Can you work these out from the model? Positions are in its coordinate system, mm. A direction names the side the tool comes from. Coordinates: 2 decimals unless noted, no trailing zeros. Write each loop counter-clockwise with the first axis right and the second up, starting at its lowest first coordinate (ties: lowest second). Pieces come first, ordered by that corner, then holes. Notation, with made-up numbers: (64, 25.5) - (104, 25.5) arc R19 ccw to (104, 31.5) - close; hole circle Ø8 at (-4.75, 21). An arc over 180 degrees is marked (long way). Use one line per item in the form item = value. Start each with the question number.
(1) If I drill on probe 1 along X at (y, z) = (2.5, 23.5); probe 2 along Z at (x, y) = (-22, 1.6); probe 3 along Z at (x, y) = (4, 2.45), over which ranges is the centre line in solid material (lowest first)? Write a range as from..to.
(2) If we section it at B-B on x = 8.5: Please give me the cut outline in (y, z).
(3) Thinking about a two-plate mould opening in Z: for faces 6 (the face through (49.603, 1, -35)), 7 (the face through (26.067, 1, -4)), 8 (the face through (44.603, 1, -5)), 9 (the face through (-9, 1, 26.568)), which applies, pulls with the +Z half, pulls with the -Z half, needs draft (parallel to the pull), parting line crosses it, or undercut?
(4) If we section it at C-C on y = 1.05: Give the number of separate pieces and of enclosed holes in the cut face, then the cut area to 3 significant figures.
(5) If we section it at A-A on z = 5.5: Please give me the cut outline in (x, y), then the cut area to 3 significant figures.
(6) For pin 1 Ø1.6 at (y, z) = (3, 0.5) entering from -X; pin 2 Ø1.5 at (y, z) = (1, 2) entering from -X; pin 3 Ø2 at (x, y) = (-2, 3) entering from +Z; pin 4 Ø10 at (x, z) = (-12.5, -22.5) entering from +Y, each with a flat end and sliding along its axis, tell me the tip position at first contact or that it passes through.
(7) On a 3-axis mill with a long thin cutter (end or side, diameter ignored), from which of +Z, -Z, +X, -X, +Y, -Y can I reach the whole of each face in a straight line? I mean faces 1 (the face through (-58.397, 1, 28)), 2 (the face through (19.273, 2.986, 18.142)), 3 (the face through (-58.397, 1, -37)), 4 (the face through (32.115, 1.479, -25.266)), 5 (the face through (-21, 1, -30.432)). Say none if no direction works.
```python
from build123d import *

# Parameters (mm, degrees)
CROQUIS2_R              = 1.5875
SALIENTE_EXTRUIR1_DEPTH = 4
CROQUIS3_W              = 6.440041964
CROQUIS3_H              = 2.682034213
CROQUIS3_W_2            = 39.119916072
CORTAR_EXTRUIR1_DEPTH   = 92
REDONDEO1_R             = 1


with BuildPart() as part:
    # Croquis2 → Saliente-Extruir1 (new body)
    with BuildSketch(Plane(origin=(0, 0, 0), x_dir=(1, 0, 0), z_dir=(0, 1, 0))):
        with BuildLine():
            Line((44.603152988, 28.432107171), (44.603152988, -19.567892829))
            ThreePointArc((44.603152988, -19.567892829), (45.188939426, -20.982106391), (46.603152988, -21.567892829))
            Line((46.603152988, -21.567892829), (47.603152988, -21.567892829))
            ThreePointArc((47.603152988, -21.567892829), (49.01736655, -22.153679266), (49.603152988, -23.567892829))
            Line((49.603152988, -23.567892829), (49.603152988, -29.567892829))
            ThreePointArc((49.603152988, -29.567892829), (49.01736655, -30.982106391), (47.603152988, -31.567892829))
            Line((47.603152988, -31.567892829), (41.603152988, -31.567892829))
            ThreePointArc((41.603152988, -31.567892829), (40.188939426, -30.982106391), (39.603152988, -29.567892829))
            Line((39.603152988, -29.567892829), (39.603152988, -29.067892829))
            Line((39.603152988, -29.067892829), (39.603152988, -26.567892829))
            Line((39.603152988, -26.567892829), (-58.396847012, -26.567892829))
            Line((-58.396847012, -26.567892829), (-58.396847012, -29.067892829))
            Line((-58.396847012, -29.067892829), (-58.396847012, -29.567892829))
            ThreePointArc((-58.396847012, -29.567892829), (-58.98263345, -30.982106391), (-60.396847012, -31.567892829))
            Line((-60.396847012, -31.567892829), (-66.396847012, -31.567892829))
            ThreePointArc((-66.396847012, -31.567892829), (-67.811060574, -30.982106391), (-68.396847012, -29.567892829))
            Line((-68.396847012, -29.567892829), (-68.396847012, -23.567892829))
            ThreePointArc((-68.396847012, -23.567892829), (-67.811060574, -22.153679266), (-66.396847012, -21.567892829))
            Line((-66.396847012, -21.567892829), (-65.396847012, -21.567892829))
            ThreePointArc((-65.396847012, -21.567892829), (-63.98263345, -20.982106391), (-63.396847012, -19.567892829))
            Line((-63.396847012, -19.567892829), (15.776989182, -19.567892829))
            ThreePointArc((15.776989182, -19.567892829), (19.312523088, -18.103426735), (20.776989182, -14.567892829))
            Line((20.776989182, -14.567892829), (20.776989182, 23.432107171))
            ThreePointArc((20.776989182, 23.432107171), (19.312523088, 26.967641077), (15.776989182, 28.432107171))
            Line((15.776989182, 28.432107171), (-63.396847012, 28.432107171))
            ThreePointArc((-63.396847012, 28.432107171), (-63.98263345, 29.846320734), (-65.396847012, 30.432107171))
            Line((-65.396847012, 30.432107171), (-66.396847012, 30.432107171))
            ThreePointArc((-66.396847012, 30.432107171), (-67.811060574, 31.017893609), (-68.396847012, 32.432107171))
            Line((-68.396847012, 32.432107171), (-68.396847012, 38.432107171))
            ThreePointArc((-68.396847012, 38.432107171), (-67.811060574, 39.846320734), (-66.396847012, 40.432107171))
            Line((-66.396847012, 40.432107171), (-60.396847012, 40.432107171))
            ThreePointArc((-60.396847012, 40.432107171), (-58.98263345, 39.846320734), (-58.396847012, 38.432107171))
            Line((-58.396847012, 38.432107171), (-58.396847012, 37.932107171))
            Line((-58.396847012, 37.932107171), (-58.396847012, 35.432107171))
            Line((-58.396847012, 35.432107171), (39.603152988, 35.432107171))
            Line((39.603152988, 35.432107171), (39.603152988, 37.932107171))
            Line((39.603152988, 37.932107171), (39.603152988, 38.432107171))
            ThreePointArc((39.603152988, 38.432107171), (40.188939426, 39.846320734), (41.603152988, 40.432107171))
            Line((41.603152988, 40.432107171), (47.603152988, 40.432107171))
            ThreePointArc((47.603152988, 40.432107171), (49.01736655, 39.846320734), (49.603152988, 38.432107171))
            Line((49.603152988, 38.432107171), (49.603152988, 32.432107171))
            ThreePointArc((49.603152988, 32.432107171), (49.01736655, 31.017893609), (47.603152988, 30.432107171))
            Line((47.603152988, 30.432107171), (46.603152988, 30.432107171))
            ThreePointArc((46.603152988, 30.432107171), (45.188939426, 29.846320734), (44.603152988, 28.432107171))
        make_face()
        with Locations(Location((-58.396847012, 32.432107171, 0), (0, 0, 270))):
            Circle(CROQUIS2_R, mode=Mode.SUBTRACT)
        with Locations(Location((-58.396847012, -23.567892829, 0), (0, 0, 270))):
            Circle(CROQUIS2_R, mode=Mode.SUBTRACT)
        with Locations(Location((39.603152988, -23.567892829, 0), (0, 0, 270))):
            Circle(CROQUIS2_R, mode=Mode.SUBTRACT)
        with Locations(Location((39.603152988, 32.432107171, 0), (0, 0, 270))):
            Circle(CROQUIS2_R, mode=Mode.SUBTRACT)
        with BuildLine():
            Line((38.434260776, 19.08388734), (38.434260776, -10.219672997))
            ThreePointArc((38.434260776, -10.219672997), (32.250588174, -16.403345599), (26.066915572, -10.219672997))
            Line((26.066915572, -10.219672997), (26.066915572, 19.08388734))
            ThreePointArc((26.066915572, 19.08388734), (32.250588174, 25.267559942), (38.434260776, 19.08388734))
        make_face(mode=Mode.SUBTRACT)
    extrude(amount=SALIENTE_EXTRUIR1_DEPTH)

    # Croquis3 → Cortar-Extruir1 (cut)
    with BuildSketch(Plane.ZY.offset(68.396847012)):
        with Locations((-27.212086189, 0.658982893)):
            Rectangle(CROQUIS3_W, CROQUIS3_H)
        with Locations((-4.432107171, 0.658982893)):
            Rectangle(CROQUIS3_W_2, CROQUIS3_H)
        with Locations((18.347871847, 0.658982893)):
            Rectangle(CROQUIS3_W, CROQUIS3_H)
    extrude(amount=-CORTAR_EXTRUIR1_DEPTH, mode=Mode.SUBTRACT)

    # Redondeo1
    redondeo1_edges = [part.edges().sort_by_distance(p)[0] for p in [
        (-9.396847012, 4, 26.567892829),
        (39.603152988, 4, 28.067892829),
        (40.188939426, 4, 30.982106391),
        (44.603152988, 4, 31.567892829),
        (49.01736655, 4, 30.982106391),
        (49.603152988, 4, 26.567892829),
        (49.01736655, 4, 22.153679266),
        (47.103152988, 4, 21.567892829),
        (45.188939426, 4, 20.982106391),
        (44.603152988, 4, -4.432107171),
        (45.188939426, 4, -29.846320734),
        (47.103152988, 4, -30.432107171),
        (49.01736655, 4, -31.017893609),
        (49.603152988, 4, -35.432107171),
        (49.01736655, 4, -39.846320734),
        (44.603152988, 4, -40.432107171),
        (40.188939426, 4, -39.846320734),
        (39.603152988, 4, -36.932107171),
        (-9.396847012, 4, -35.432107171),
        (-58.396847012, 4, -36.932107171),
        (-58.98263345, 4, -39.846320734),
        (-63.396847012, 4, -40.432107171),
        (-67.811060574, 4, -39.846320734),
        (-68.396847012, 4, -35.432107171),
        (-67.811060574, 4, -31.017893609),
        (-65.896847012, 4, -30.432107171),
        (-63.98263345, 4, -29.846320734),
        (32.250588174, 4, 16.403345599),
        (26.066915572, 4, -4.432107171),
        (32.250588174, 4, -25.267559942),
        (38.434260776, 4, -4.432107171),
        (-63.98263345, 4, 20.982106391),
        (-65.896847012, 4, 21.567892829),
        (-67.811060574, 4, 22.153679266),
        (-68.396847012, 4, 26.567892829),
        (-67.811060574, 4, 30.982106391),
        (-63.396847012, 4, 31.567892829),
        (-58.98263345, 4, 30.982106391),
        (-58.396847012, 4, 28.067892829),
    ]]
    fillet(redondeo1_edges, radius=REDONDEO1_R)


solid = part.part
```
Reported:
q1.probe_1 = -68.4..-59.98, -56.81..38.02, 41.19..49.6
q1.probe_2 = -35.43..-30.43, 21.57..26.57
q1.probe_3 = -35.43..-28.43, 19.57..26.57
q2.outline = (0, -35.43) - (3, -35.43) arc R1 ccw to (4, -34.43) - (4, -28.43) - (2, -28.43) - (2, -30.43) - (0, -30.43) - close; (0, 21.57) - (2, 21.57) - (2, 19.57) - (4, 19.57) - (4, 25.57) arc R1 ccw to (3, 26.57) - (0, 26.57) - close
q3.face_6 = needs draft
q3.face_7 = undercut
q3.face_8 = undercut
q3.face_9 = pulls with the +Z half
q4.separate_pieces = 1
q4.enclosed_holes = 5
q4.area = 1,950 mm2
q5.outline = (20.78, 2) - (23.6, 2) - (23.6, 0) - (26.07, 0) - (26.07, 3) arc R1 ccw to (25.07, 4) - (20.78, 4) - close; (38.43, 0) - (44.6, 0) - (44.6, 3) arc R1 ccw to (43.6, 4) - (39.43, 4) arc R1 ccw to (38.43, 3) - close
q5.area = 39.5 mm2
q6.pin_1 = 20.78
q6.pin_2 = 23.6
q6.pin_3 = 26.57
q6.pin_4 = through
q7.face_1 = +Z, +Y, -Y
q7.face_2 = -X, +Y, -Y
q7.face_3 = -Z, +Y, -Y
q7.face_4 = +Y, -Y
q7.face_5 = -X, -Y
